Can you work these out from the model? Positions are in its coordinate system, mm. Face numbers are marked on the shaded views. A direction names the side the tool comes from. Give positions to 0.01 mm unless a question says otherwise; leave off trailing zeros. Order: outer loops, then holes, each group sorted by start corner. A loop starts at its lowest first (then second) coordinate and runs counter-clockwise, first axis right, second up.
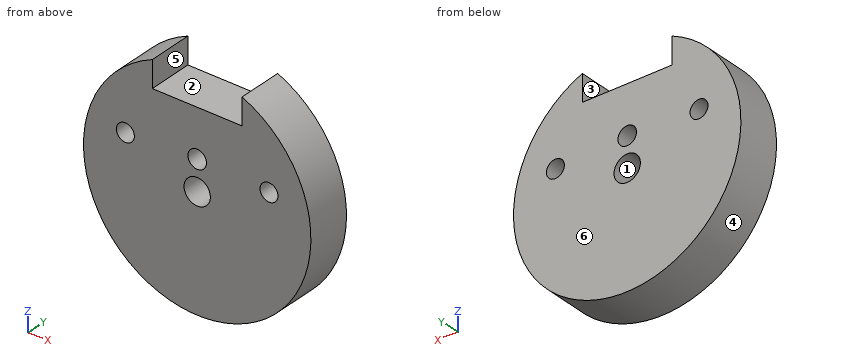
```python
from build123d import *

# Parameters (mm, degrees)
SKETCH1_R              = 3.81
SKETCH1_R_2            = 3.937
SKETCH1_R_3            = 5.588
BOSS_EXTRUDE1_DEPTH    = 19.05
SKETCH2_W              = 175.508996812
SKETCH2_H              = 124.727535594
SKETCH2_R              = 48.26
TOLERANCE_ADJUST_DEPTH = 63.5


with BuildPart() as part:
    # Sketch1 → Boss-Extrude1 (new body)
    with BuildSketch(Plane(origin=(0, 0, 0), x_dir=(1, 0, 0), z_dir=(0, 1, 0))):
        with BuildLine():
            Line((-19.05, -33.02), (19.05, -33.02))
            Line((19.05, -33.02), (19.05, -45.72))
            ThreePointArc((19.05, -45.72), (41.211451079, -27.474300719), (49.53, 0))
            ThreePointArc((49.53, 0), (-27.474300719, 41.211451079), (-19.05, -45.72))
            Line((-19.05, -45.72), (-19.05, -33.02))
        make_face()
        with Locations(Location((-30.48, -11.43, 0), (0, 0, 90))):
            Circle(SKETCH1_R, mode=Mode.SUBTRACT)
        with Locations(Location((0, -12.7, 0), (0, 0, 90))):
            Circle(SKETCH1_R_2, mode=Mode.SUBTRACT)
        with Locations(Location((30.48, -11.43, 0), (0, 0, 90))):
            Circle(SKETCH1_R, mode=Mode.SUBTRACT)
        with Locations(Location((0, 0, 0), (0, 0, 90))):
            Circle(SKETCH1_R_3, mode=Mode.SUBTRACT)
    extrude(amount=BOSS_EXTRUDE1_DEPTH)

    # Sketch2 → Tolerance Adjust (cut)
    with BuildSketch(Plane(origin=(0, 0, 0), x_dir=(1, 0, 0), z_dir=(0, 1, 0))):
        Rectangle(SKETCH2_W, SKETCH2_H)
        Circle(SKETCH2_R, mode=Mode.SUBTRACT)
    extrude(amount=TOLERANCE_ADJUST_DEPTH, mode=Mode.SUBTRACT)


solid = part.part
```
1) Suppose I cut it at B-B (x = 32). Please give me the cut outline in (y, z), and give its area (3 significant figures).
2) I'm going to push flat-ended pins straight in: pin 1 Ø2 at (y, z) = (11, -5.5) entering from +X; pin 2 Ø1.5 at (x, y) = (36.5, 8) entering from +Z; pin 3 Ø4 at (x, y) = (11, 14.5) entering from -Z. Where does each tip first touch, or does it pass through?
3) We'd pull the mould along X, two halves only. Please class the marked faces 3, 4, 5 and 6: +X half, -X half, draft (parallel to the pull), parting line (faces both ways), or undercut.
4) Suppose I cut it at D-D (z = 11.43). Please give me the cut outline in (x, y), and give its area (3 significant figures).
5) If I drill on line 1 (X direction, y = 6, z = 11.43); line 2 (Z direction, x = 34, y = 17.5); line 3 (Z direction, x = 30.48, y = 5.75), over which ranges is the centre line in solid material (lowest first)?
6) Suppose I cut it at A-A (y = 6.5). Please give me the cut outline in (x, z), and give its area (3 significant figures).
7) Which directions (+Z, -Z, +X, -X, +Y, -Y) give clear straight access to the entire face, cutting with the end or side of a thin tool? Please do the marked faces 1 and 2.
8) Suppose I cut it at C-C (z = 38). Please give me the cut outline in (x, y), and give its area (3 significant figures).
Results:
1. outline: (0, -36.13) - (19.05, -36.13) - (19.05, 7.94) - (0, 7.94) - close; (0, 14.92) - (19.05, 14.92) - (19.05, 36.13) - (0, 36.13) - close
1. area: 1,240 mm2
2. pin 1: stops at x = 48.05
2. pin 2: stops at z = 32.42
2. pin 3: stops at z = -47.41
3. face 3: undercut
3. face 4: parting line
3. face 5: undercut
3. face 6: draft
4. outline: (-46.89, 0) - (-34.29, 0) - (-34.29, 19.05) - (-46.89, 19.05) - close; (-26.67, 0) - (-3.73, 0) - (-3.73, 19.05) - (-26.67, 19.05) - close; (3.73, 0) - (26.67, 0) - (26.67, 19.05) - (3.73, 19.05) - close; (34.29, 0) - (46.89, 0) - (46.89, 19.05) - (34.29, 19.05) - close
4. area: 1,350 mm2
5. line 1: x = -46.89 to -34.29, -26.67 to -3.73, 3.73 to 26.67, 34.29 to 46.89
5. line 2: z = -34.25 to 9.97, 12.89 to 34.25
5. line 3: z = -37.42 to 7.62, 15.24 to 37.42
6. outline: (-19.05, 33.02) - (-19.05, 44.34) arc R48.26 ccw (long way) to (19.05, 44.34) - (19.05, 33.02) - close; hole circle Ø7.62 at (-30.48, 11.43); hole circle Ø11.18 at (0, 0); hole circle Ø7.87 at (0, 12.7); hole circle Ø7.62 at (30.48, 11.43)
6. area: 6,550 mm2
7. face 1: +Y, -Y
7. face 2: +Z, +Y, -Y
8. outline: (-29.75, 0) - (-19.05, 0) - (-19.05, 19.05) - (-29.75, 19.05) - close; (19.05, 0) - (29.75, 0) - (29.75, 19.05) - (19.05, 19.05) - close
8. area: 408 mm2
